```python
from build123d import *

# Parameters (mm, degrees)
SKETCH1_R           = 3.96875
SKETCH1_R_2         = 2
BOSS_EXTRUDE1_DEPTH = 3.175


with BuildPart() as part:
    # Sketch1 → Boss-Extrude1 (new body)
    with BuildSketch(Plane(origin=(0, 0, 0), x_dir=(1, 0, 0), z_dir=(0, 1, 0))):
        with BuildLine():
            Line((1.402094694, -6.193273001), (-25.521322666, -12.288463801))
            ThreePointArc((-25.521322666, -12.288463801), (-29.985830904, -9.750697408), (-27.867805259, -5.07244352))
            Line((-27.867805259, -5.07244352), (-2.508709628, 5.833427466))
            ThreePointArc((-2.508709628, 5.833427466), (6.03875237, 1.963662347), (1.402094694, -6.193273001))
        make_face()
        with Locations(Location((0, 0, 0), (0, 0, 270))):
            Circle(SKETCH1_R, mode=Mode.SUBTRACT)
        with Locations(Location((-26.362579482, -8.5725, 0), (0, 0, 270))):
            Circle(SKETCH1_R_2, mode=Mode.SUBTRACT)
        with BuildLine():
            Line((-4.113361585, -4.837639556), (-21.927586713, -8.870600886))
            ThreePointArc((-21.927586713, -8.870600886), (-22.135452823, -7.197936357), (-22.951139301, -5.722920928))
            Line((-22.951139301, -5.722920928), (-6.17196775, 1.493088778))
            ThreePointArc((-6.17196775, 1.493088778), (-6.03875237, -1.963662347), (-4.113361585, -4.837639556))
        make_face(mode=Mode.SUBTRACT)
    extrude(amount=-BOSS_EXTRUDE1_DEPTH)


solid = part.part
```
The model under review builds one solid part; all positions refer to its coordinate system, in mm. A direction names the side the tool comes from. Round coordinates to 2 decimals unless told otherwise and drop trailing zeros. Write each loop counter-clockwise with the first axis right and the second up, starting at its lowest first coordinate (ties: lowest second). Pieces come first, ordered by that corner, then holes.
(1) Mouldability with a two-part tool opening along Z and no side actions: class faces 3 (the flat face through (-14.679, -1.565, 2.165)), 4 (the cylindrical face through (5.991, -1.565, -2.104)), 5 (the flat face through (-15.366, -1.565, -0.304)) as +Z half, -Z half, draft (parallel to the pull), parting line (faces both ways), or undercut.
(2) We need section D-D on z = 9.25. Give the boundary of the cut face in (x, y) (3 decimals).
(3) Machinability: for faces 1 (the flat face through (-12.896, -1.565, 6.826)), 2 (the flat face through (-10.5, -3.175, 0.2)), which of the approach directions +Z, -Z, +X, -X, +Y, -Y give a long, thin tool a straight path to every point of the face, cutting with its end or side? Answer none if there is none.
(4) Insertion check: pin 1 (6 mm diameter, centred on x = -12, z = -3.5, fed in from +Y); pin 2 (1.5 mm diameter, centred on x = -2.5, y = -1.5, fed in from -Z). Each pin has a flat end and moves straight along its axis. Give the tip position at first contact, or say it passes through.
(5) We need section C-C on y = -2.45. Give the number of separate pieces and of enclosed holes in the cut face, and give its area (3 significant figures).
(6) Wall thickness on L1, parallel to X at y = -1, z = 0; L2, parallel to X at y = -2.6, z = 2.25; L3, parallel to Z at x = -2.5, y = -0.75: over which ranges is each line inside the solid? List them lowest first.
(7) We need section A-A on z = 0. Give the boundary of the cut face in (x, y) (3 decimals).
(8) We need section B-B on x = 3. Give the boundary of the cut face in (y, z) (3 decimals), and give its area (3 significant figures).
Findings below:
1. face 3: undercut
1. face 4: parting line
1. face 5: -Z half
2. outline: (-30.112, -3.175) - (-28.244, -3.175) - (-28.244, 0) - (-30.112, 0) - close; (-24.481, -3.175) - (-12.1, -3.175) - (-12.1, 0) - (-24.481, 0) - close
3. face 1: +Y, -Y
3. face 2: +Z, -Z, +X, -X, -Y
4. pin 1: stops at y = 0
4. pin 2: stops at z = -6.1
5. separate pieces: 1
5. enclosed holes: 3
5. area: 221 mm2
6. L1: x = -16.07 to -9.64, -6.35 to -3.97, 3.97 to 6.35
6. L2: x = -21.3 to -14.88, -5.94 to -3.27, 3.27 to 5.94
6. L3: z = -5.84 to -3.08, 3.08 to 7.08
7. outline: (-16.073, -3.175) - (-9.644, -3.175) - (-9.644, 0) - (-16.073, 0) - close; (-6.35, -3.175) - (-3.969, -3.175) - (-3.969, 0) - (-6.35, 0) - close; (3.969, -3.175) - (6.35, -3.175) - (6.35, 0) - (3.969, 0) - close
8. outline: (-3.175, -5.597) - (0, -5.597) - (0, -2.598) - (-3.175, -2.598) - close; (-3.175, 2.598) - (0, 2.598) - (0, 5.597) - (-3.175, 5.597) - close
8. area: 19.0 mm2
